```python
from build123d import *

# Parameters (mm, degrees)
SKETCH1_R                = 18
SKETCH1_R_2              = 8
BOSS_EXTRUDE1_DEPTH      = 3
SKETCH2_R                = 11
SKETCH2_R_2              = 8
BOSS_EXTRUDE2_DEPTH      = 22
M_0_295_DIAMETER_HOLE1_D = 3.099999896
BOSS_EXTRUDE3_DEPTH      = 1.5
CIRPATTERN1_COUNT        = 6
CHAMFER2_SIZE            = 0.5
SKETCH6_R                = 11
BOSS_EXTRUDE4_DEPTH      = 3
SKETCH8_R                = 8
BOSS_EXTRUDE5_DEPTH      = 2
CHAMFER3_SIZE            = 6
SKETCH7_R                = 2.4
CUT_EXTRUDE1_DEPTH       = 2
CUT_EXTRUDE2_REACH       = 28
SKETCH9_R                = 1.05
SKETCH10_R               = 11
SKETCH10_R_2             = 10
CUT_EXTRUDE3_DEPTH       = 12
CHAMFER4_SIZE            = 0.5
CHAMFER5_SIZE            = 2
CHAMFER5_SIZE2           = 3.464101615


with BuildPart() as part:
    # Sketch1 → Boss-Extrude1 (new body)
    with BuildSketch(Plane(origin=(0, 0, 0), x_dir=(1, 0, 0), z_dir=(0, 1, 0))):
        Circle(SKETCH1_R)
        Circle(SKETCH1_R_2, mode=Mode.SUBTRACT)
    extrude(amount=BOSS_EXTRUDE1_DEPTH)

    # Sketch2 → Boss-Extrude2 (add)
    with BuildSketch(Plane(origin=(0, 3, 0), x_dir=(1, 0, 0), z_dir=(0, 1, 0))):
        Circle(SKETCH2_R)
        Circle(SKETCH2_R_2, mode=Mode.SUBTRACT)
    extrude(amount=BOSS_EXTRUDE2_DEPTH)

    # M (0.295) Diameter Hole1 (through all)
    with Locations(Plane(origin=(0, 3, 14.5), x_dir=(0, 0, 1), z_dir=(0, 1, 0))):
        with Locations((0, 0), (-7.25, -12.557368355), (-7.25, 12.557368355), (-21.75, 12.557368355), (-29, 0), (-21.75, -12.557368355)):
            Hole(M_0_295_DIAMETER_HOLE1_D / 2)

    # Sketch5 → Boss-Extrude3 (add, symmetric)
    with BuildSketch(Plane.XY):
        Polygon((11, 13), (17, 4.428571429), (17, 3), (17, 2.5), (10.5, 2.5), (10.5, 13), align=None)
    boss_extrude3 = extrude(amount=BOSS_EXTRUDE3_DEPTH, both=True)

    # CirPattern1: Boss-Extrude3 ×6 about axis
    cirpattern1_axis = Axis((0, 0, 0), (0, 1, 0))
    for i in range(1, CIRPATTERN1_COUNT):
        add(boss_extrude3.rotate(cirpattern1_axis, i * 360 / CIRPATTERN1_COUNT))

    # Chamfer2
    chamfer2_edges = [part.edges().sort_by_distance(p)[0] for p in [
        (-18, 3, 0),
    ]]
    chamfer(chamfer2_edges, length=CHAMFER2_SIZE)

    # Sketch6 → Boss-Extrude4 (add)
    with BuildSketch(Plane(origin=(0, 25, 0), x_dir=(1, 0, 0), z_dir=(0, 1, 0))):
        Circle(SKETCH6_R)
    extrude(amount=BOSS_EXTRUDE4_DEPTH)

    # Sketch8 → Boss-Extrude5 (add)
    with BuildSketch(Plane.XZ.offset(-25)):
        Circle(SKETCH8_R)
    extrude(amount=BOSS_EXTRUDE5_DEPTH)

    # Chamfer3
    chamfer3_edges = [part.edges().sort_by_distance(p)[0] for p in [
        (-11, 28, 0),
    ]]
    chamfer(chamfer3_edges, length=CHAMFER3_SIZE)

    # Sketch7 → Cut-Extrude1 (cut)
    with BuildSketch(Plane(origin=(0, 28, 0), x_dir=(1, 0, 0), z_dir=(0, 1, 0))):
        Circle(SKETCH7_R)
    extrude(amount=-CUT_EXTRUDE1_DEPTH, mode=Mode.SUBTRACT)

    # Sketch9 → Cut-Extrude2 (cut, up to next)
    with BuildSketch(Plane(origin=(0, 26, 0), x_dir=(1, 0, 0), z_dir=(0, 1, 0)), mode=Mode.PRIVATE) as cut_extrude2_sk1:
        Circle(SKETCH9_R)
    cut_extrude2_tool1 = extrude(cut_extrude2_sk1.sketch, amount=-CUT_EXTRUDE2_REACH, mode=Mode.PRIVATE) & part.part
    add(cut_extrude2_tool1.solids().sort_by_distance((0, 26, 0))[0], mode=Mode.SUBTRACT)

    # Sketch10 → Cut-Extrude3 (cut)
    with BuildSketch(Plane(origin=(0, 28, 0), x_dir=(1, 0, 0), z_dir=(0, 1, 0))):
        Circle(SKETCH10_R)
        Circle(SKETCH10_R_2, mode=Mode.SUBTRACT)
    extrude(amount=-CUT_EXTRUDE3_DEPTH, mode=Mode.SUBTRACT)

    # Chamfer4
    chamfer4_edges = [part.edges().sort_by_distance(p)[0] for p in [
        (-11, 16, 0),
    ]]
    chamfer(chamfer4_edges, length=CHAMFER4_SIZE)

    # Sketch11 → Cut-Revolve1 (revolve, cut)
    with BuildSketch(Plane.XY):
        Polygon((-5, 28), (-5, 29.257596247), (-10, 29.257596247), (-10, 23), (-5.989740888, 25.017543101), align=None)
    revolve(axis=Axis((0, 18, 0), (0, -1, 0)), mode=Mode.SUBTRACT)

    # Chamfer5
    chamfer5_edges = [part.edges().sort_by_distance(p)[0] for p in [
        (-8, 23, 0),
    ]]
    chamfer5_side = [part.faces().sort_by_distance(p)[0] for p in [
        (-8, 11.5, 0),
    ]]
    chamfer(chamfer5_edges, length=CHAMFER5_SIZE, length2=CHAMFER5_SIZE2, reference=chamfer5_side[0])


solid = part.part
```
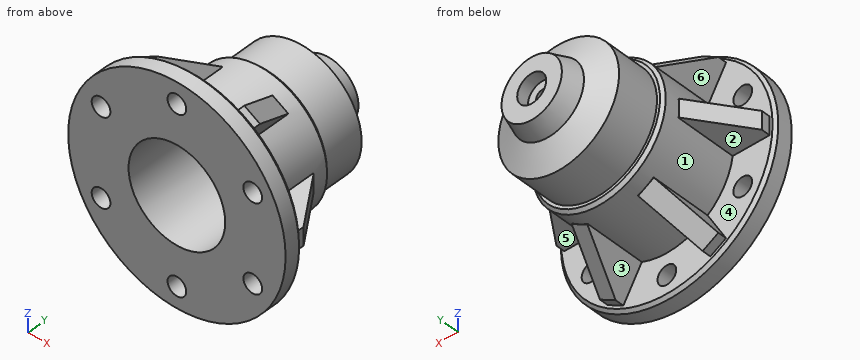
Verification items for the finished model (mm, model axes). Face numbers are marked on the shaded views. A direction names the side the tool comes from. Round coordinates to 2 decimals unless told otherwise and drop trailing zeros. Order: outer loops, then holes, each group sorted by start corner. A loop starts at its lowest first (then second) coordinate and runs counter-clockwise, first axis right, second up. Notation, with made-up numbers: (-33, 84) - (-21, 84) arc R35 ccw to (-21, 118) - close; hole circle Ø10 at (-38, -32). An arc over 180 degrees is marked (long way). Use CSV: the item, a comma, the result in double quotes.
(1) Gauge pin test, flat ends, axial feed: pin 1 Ø0.7 at (x, z) = (-6, -9) entering from +Y; pin 2 Ø0.8 at (x, z) = (-5, -10) entering from +Y; pin 3 Ø1.7 at (x, z) = (0, 0) entering from +Y; pin 4 Ø3.5 at (x, z) = (-12.56, -7.25) entering from +Y. Record the tip position at first contact, or that the pin passes through.
Entries:
pin 1,"y = 16"
pin 2,"y = 15.72"
pin 3,"through"
pin 4,"y = 3"
(2) Section check A-A on y = 12.5. Record the boundary of the cut face in (x, z), and give its area (3 significant figures).
Entries:
outline,"(-11.35, -1.5) - (-10.9, -1.5) arc R11 ccw to (-6.75, -8.69) - (-6.97, -9.08) - (-4.38, -10.58) - (-4.15, -10.19) arc R11 ccw to (4.15, -10.19) - (4.38, -10.58) - (6.97, -9.08) - (6.75, -8.69) arc R11 ccw to (10.9, -1.5) - (11.35, -1.5) - (11.35, 1.5) - (10.9, 1.5) arc R11 ccw to (6.75, 8.69) - (6.97, 9.08) - (4.38, 10.58) - (4.15, 10.19) arc R11 ccw to (-4.15, 10.19) - (-4.38, 10.58) - (-6.97, 9.08) - (-6.75, 8.69) arc R11 ccw to (-10.9, 1.5) - (-11.35, 1.5) - close; hole circle Ø16 at (0, 0)"
area,"186 mm^2"
(3) Section check B-B on x = 0. State how many separate pieces and enclosed holes the cut face has, and give its area (3 significant figures).
Entries:
separate pieces,"4"
enclosed holes,"0"
area,"203 mm^2"
(4) Mould release check, pull along X, two halves, no side actions. Record for the marked faces 4, 5 and 6: released by +X, released by -X, zero draft, split by the parting line, or undercut.
Entries:
face 4,"undercut"
face 5,"zero draft"
face 6,"released by -X"
(5) Access from +Z, -Z, +X, -X, +Y, -Y to the whole of each face (thin tool, end or side, straight path). Record for the marked faces 1, 2 and 3.
Entries:
face 1,"+Y"
face 2,"-Z, -X, +Y"
face 3,"-Z, +Y"
(6) Thickness scan on probe 1 along Z at (x, y) = (0, 6.5); probe 2 along X at (y, z) = (2.35, 7.25); probe 3 along Y at (x, z) = (-11, 13.5). Record the ranges inside material, lowest first. Write a range as from..to.
Entries:
probe 1,"-11..-8, 8..11"
probe 2,"-16.48..-14.11, -11.01..-3.38, 3.38..11.01, 14.11..16.48"
probe 3,"0..3"
